For this review, take the finished solid that the model builds, in its own axes (mm). Face numbers are marked on the shaded views. A direction names the side the tool comes from. Coordinates: 2 decimals unless noted, no trailing zeros. Order: outer loops, then holes, each group sorted by start corner. A loop starts at its lowest first (then second) coordinate and runs counter-clockwise, first axis right, second up. Notation, with made-up numbers: (75, 0) -> (87, 0) arc R14 cw to (87, 24) -> close; hole circle Ø7 at (3, 0.5). An arc over 180 degrees is marked (long way). Return JSON: item names as keys, results as strings. Group by question number.
Item 1: Take a section at D-D (z = 10). Write out the cut boundary in (x, y) (3 decimals).
Item 2: Machinability: for the marked faces 1, 2 and 3, which of the approach directions +Z, -Z, +X, -X, +Y, -Y give a long, thin tool a straight path to every point of the face, cutting with its end or side? Answer none if there is none.
Item 3: For line 1 along Y through (x, z) = (0, 9.3) (3 decimals); line 2 along Y through (x, z) = (0, 10.9) (3 decimals); line 3 along X through (y, z) = (0.5, 9.25), list the stretches that pass through material, from the lowest coordinate up.
Item 4: Take a section at B-B (z = 4.75). Write out the cut boundary in (x, y) (3 decimals), then the cut area to 3 significant figures.
Item 5: Draft analysis for pull direction X (two halves, no side actions). For the marked faces 4, 5 and 6, state which applies: +X half, -X half, draft (parallel to the pull), parting line (faces both ways), or undercut.
Item 6: Insertion check: pin 1 (8 mm diameter, centred on x = -6, y = 9, fed in from -Z); pin 2 (10 mm diameter, centred on y = -7.5, z = 7, fed in from +X); pin 3 (4 mm diameter, centred on y = -4, z = 6.5, fed in from +X); pin 4 (10 mm diameter, centred on x = -0.5, z = 10, fed in from +Y). Each pin has a flat end and moves straight along its axis. Give the tip position at first contact, or say it passes through.
Item 7: Take a section at A-A (y = 0). Write out the cut boundary in (x, z) (3 decimals), then the cut area to 3 significant figures.
Autodesk Inventor part; units mm, degrees
ref_plane "YZ Plane" through (0, 0, 0) normal (1, 0, 0) x (0, 1, 0)
ref_plane "XZ Plane" through (0, 0, 0) normal (0, 1, 0) x (-1, 0, 0)
ref_plane "XY Plane" through (0, 0, 0) normal (0, 0, 1) x (1, 0, 0)
sketch "Sketch1" plane through (0, 0, 0) normal (0, 0, 1) x (1, 0, 0)
  circle A0 centre (0, 0) radius 12.827
  dimension "d0" = 25.654
extrude "Extrusion1" add sketch "Sketch1" along normal blind 12.7254
sketch "Sketch2" plane through (0, 0, 12.7254) normal (0, 0, 1) x (1, 0, 0)
  circle A0 centre (0, 0) radius 9.525
  circle A1 centre (0, 0) radius 4.445
  dimension "d3" = 19.05
  dimension "d4" = 8.89
extrude "Extrusion2" cut sketch "Sketch2" against normal blind 5.715
sketch "Sketch3" plane through (0, 0, 0) normal (0, 0, -1) x (-1, 0, 0)
  circle A0 centre (0, 0) radius 4.445
  circle A1 centre (0, 0) radius 9.525
extrude "Extrusion3" cut sketch "Sketch3" against normal blind 5.715
sketch "Sketch4" plane through (0, 0, 12.7254) normal (0, 0, 1) x (1, 0, 0)
  circle A0 centre (0, 0) radius 4.445
extrude "Extrusion4" add sketch "Sketch4" along normal blind 3.1623
sketch "Sketch5" plane through (0, 0, 0) normal (0, 0, -1) x (-1, 0, 0)
  circle A0 centre (0, 0) radius 4.445
extrude "Extrusion5" add sketch "Sketch5" along normal blind 3.1623
fillet "Fillet1" radius 3.175 2 edges at (-12.827, 0, 12.7254) (-12.827, 0, 0)
properties part number "CastorWheel" material "ABS Plastic"
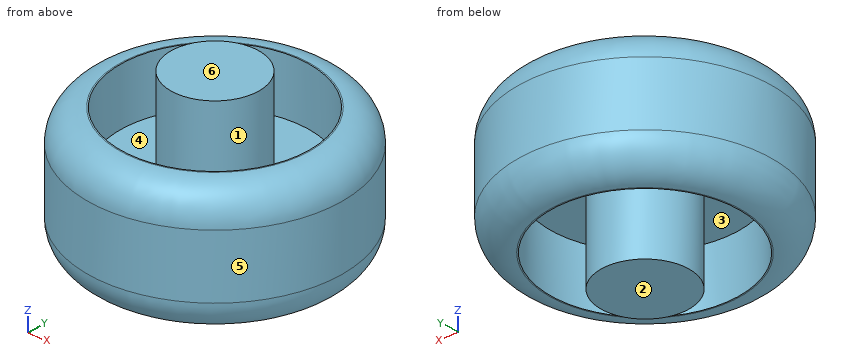
Findings below:
{
 "1": {"outline": "circle Ø25.59 at (0, 0); circle Ø8.89 at (0, 0); hole circle Ø19.05 at (0, 0)"},
 "2": {"face 1": "+Z", "face 2": "-Z, +X, -X, +Y, -Y", "face 3": "-Z"},
 "3": {"line 1": "y = -12.827 to -9.525, -4.445 to 4.445, 9.525 to 12.827", "line 2": "y = -12.526 to -9.525, -4.445 to 4.445, 9.525 to 12.526", "line 3": "x = -12.82 to -9.51, -4.42 to 4.42, 9.51 to 12.82"},
 "4": {"outline": "circle Ø25.654 at (0, 0); circle Ø8.89 at (0, 0); hole circle Ø19.05 at (0, 0)", "area": "294 mm2"},
 "5": {"face 4": "undercut", "face 5": "parting line", "face 6": "draft"},
 "6": {"pin 1": "stops at z = 0", "pin 2": "stops at x = 12.58", "pin 3": "stops at x = 12.67", "pin 4": "stops at y = 12.83"},
 "7": {"outline": "(-12.827, 3.175) arc R3.175 ccw to (-9.652, 0) -> (-9.525, 0) -> (-9.525, 5.715) -> (-4.445, 5.715) -> (-4.445, -3.162) -> (4.445, -3.162) -> (4.445, 5.715) -> (9.525, 5.715) -> (9.525, 0) -> (9.652, 0) arc R3.175 ccw to (12.827, 3.175) -> (12.827, 9.55) arc R3.175 ccw to (9.652, 12.725) -> (9.525, 12.725) -> (9.525, 7.01) -> (4.445, 7.01) -> (4.445, 15.888) -> (-4.445, 15.888) -> (-4.445, 7.01) -> (-9.525, 7.01) -> (-9.525, 12.725) -> (-9.652, 12.725) arc R3.175 ccw to (-12.827, 9.55) -> close", "area": "258 mm2"}
}
